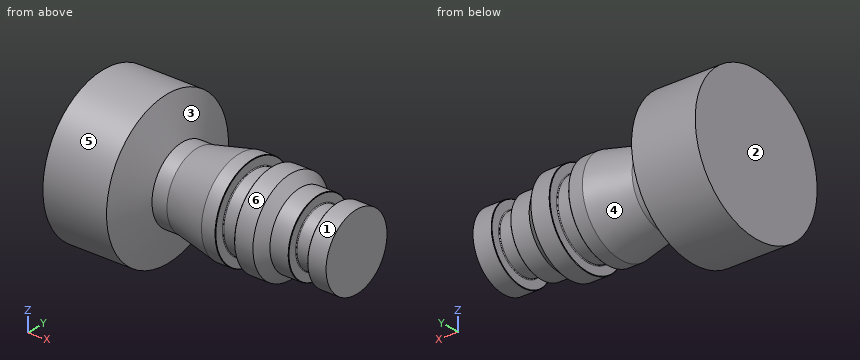
from build123d import *

# Parameters (mm, degrees)
CHAMFER1_SIZE = 0.3048


with BuildPart() as part:
    # Sketch1 → Base-Revolve (revolve)
    with BuildSketch(Plane.XY, mode=Mode.PRIVATE) as base_revolve_sk:
        with BuildLine():
            Line((0, 0), (0, 25.4))
            Line((0, 25.4), (-12.7, 25.4))
            Line((-12.7, 25.4), (-12.7, 19.558))
            ThreePointArc((-12.7, 19.558), (-12.848789755, 19.198789755), (-13.208, 19.05))
            Line((-13.208, 19.05), (-24.892, 19.05))
            ThreePointArc((-24.892, 19.05), (-25.251210245, 19.198789755), (-25.4, 19.558))
            Line((-25.4, 19.558), (-25.4, 25.4))
            Line((-25.4, 25.4), (-38.1, 25.4))
            Line((-38.1, 25.4), (-44.45, 31.75))
            Line((-44.45, 31.75), (-57.15, 31.75))
            Line((-57.15, 31.75), (-57.15, 25.908))
            ThreePointArc((-57.15, 25.908), (-57.298789755, 25.548789755), (-57.658, 25.4))
            Line((-57.658, 25.4), (-69.342, 25.4))
            ThreePointArc((-69.342, 25.4), (-69.701210245, 25.548789755), (-69.85, 25.908))
            Line((-69.85, 25.908), (-69.85, 31.75))
            Line((-69.85, 31.75), (-79.375, 31.75))
            Line((-79.375, 31.75), (-107.95, 25.4))
            Line((-107.95, 25.4), (-118.11, 25.4))
            Line((-118.11, 25.4), (-128.27, 50.8))
            Line((-128.27, 50.8), (-171.45, 50.8))
            Line((-171.45, 50.8), (-171.45, 0))
            Line((-171.45, 0), (0, 0))
        make_face()
    revolve(base_revolve_sk.sketch.rotate(Axis((0, 0, 0), (-1, 0, 0)), 90), axis=Axis((0, 0, 0), (-1, 0, 0)))

    # Chamfer1
    chamfer1_edges = [part.edges().sort_by_distance(p)[0] for p in [
        (-12.7, 0, 25.4),
        (-25.4, 0, 25.4),
        (-57.15, 0, 31.75),
        (-69.85, 0, 31.75),
    ]]
    chamfer(chamfer1_edges, length=CHAMFER1_SIZE)


solid = part.part
CAD build for the part. Positions are in the model's coordinates, mm. Face numbers are marked on the shaded views. A direction names the side the tool comes from. Give positions to 0.01 mm unless a question says otherwise; leave off trailing zeros. Loops run counter-clockwise (first coordinate to the right, second up) from the corner with the lowest first, then second, coordinate; pieces in that order, holes last. Notation, with made-up numbers: M 0,-35 L 18,-35 A26 cw 18,-7 Z; hole C 22.25,56 d7. An arc over 180 degrees is marked long. Answer in a Markdown table with one row per item. Add a question column.
Item 1: Probe probe 1 along X at (y, z) = (-20.5, 2.5); probe 2 along Y at (x, z) = (-32.5, -4); probe 3 along Z at (x, y) = (-79, 1). List the from-to ranges inside material, lowest first.
Item 2: Tool access for the marked faces 4, 5 and 6: list every direction of +Z, -Z, +X, -X, +Y, -Y with a clear straight run to the whole face (end or side of a thin tool).
Item 3: Band-saw the part on B-B on x = -151.5. Give the cut face in (y, z).
Item 4: Band-saw the part on A-A on x = -116. Give the cut face in (y, z).
Item 5: Mould opens along X. For the marked faces 1, 2 and 3 say: +X half, -X half, draft (parallel to the pull), parting line (faces both ways), or undercut.
Item 6: Drop flat-ended pins along their axis: P1, Ø1, axis at x = -60.5, z = 21.5, coming from the -Y side; P2, Ø5, axis at x = -62, z = -25, coming from the -Y side; P3, Ø8, axis at y = 34, z = -33, coming from the +X side. Give the stop position or say it passes through.
Reply:
| question | item | result |
|---|---|---|
| 1 | probe 1 | x = -171.45 to -25.4, -12.7 to 0 |
| 1 | probe 2 | y = -25.08 to 25.08 |
| 1 | probe 3 | z = -31.73 to 31.73 |
| 2 | face 4 | none |
| 2 | face 5 | +X, -X |
| 2 | face 6 | +X |
| 3 | outline | C 0,0 d101.6 |
| 4 | outline | C 0,0 d50.8 |
| 5 | face 1 | draft |
| 5 | face 2 | -X half |
| 5 | face 3 | undercut |
| 6 | P1 | stops at y = -14.29 |
| 6 | P2 | stops at y = -11.79 |
| 6 | P3 | stops at x = -125.3 |
